Could you check a few things on this drawing? It's one solid part, dimensions in mm from its lowest x, y, z. A direction names the side the tool comes from. Give positions to 0.01 mm unless a question says otherwise; leave off trailing zeros. Use one line per item in the form item = value.
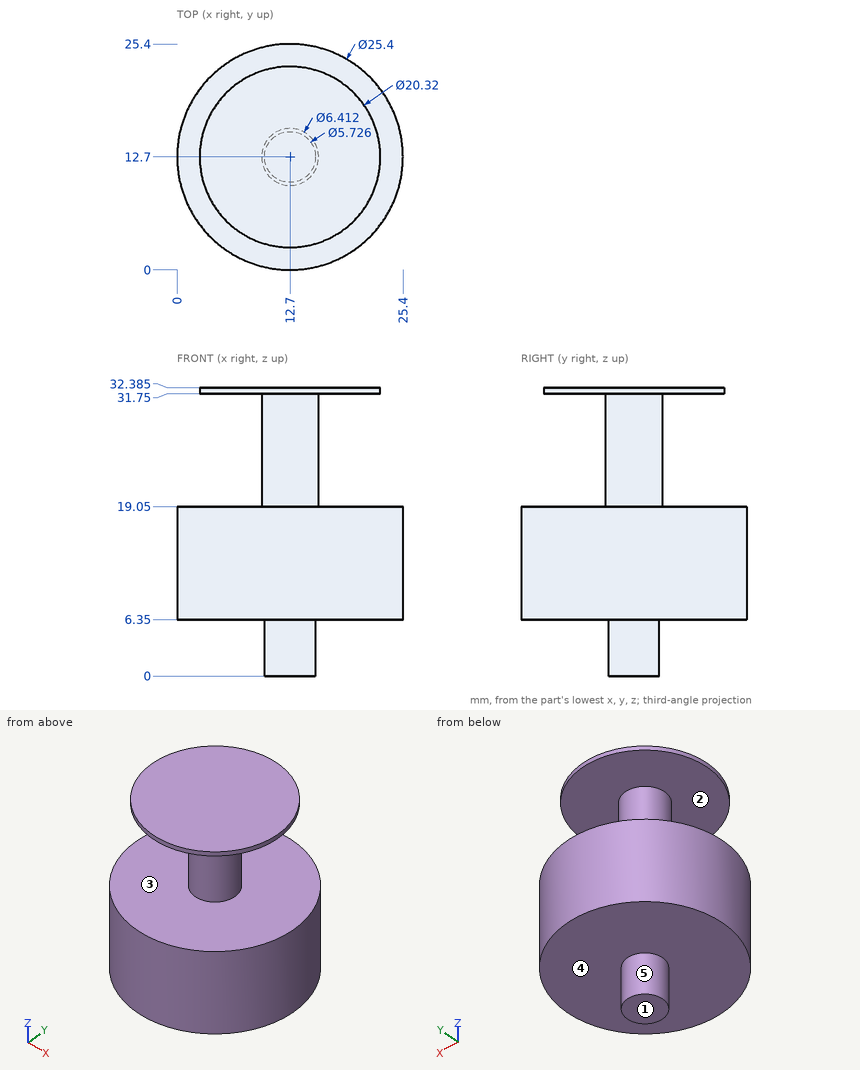
Q1. Thinking about a two-plate mould opening in Z: for the marked faces 3, 4 and 5, which applies, +Z half, -Z half, draft (parallel to the pull), parting line (faces both ways), or undercut?
Found:
face_3 = undercut
face_4 = -Z half
face_5 = draft
Q2. I'm going to push flat-ended pins straight in: pin 1 Ø1 at (y, z) = (9.5, 12.5) entering from +X; pin 2 Ø5 at (x, z) = (19, 17.5) entering from -Y; pin 3 Ø4 at (x, z) = (5, 18.5) entering from +Y. Where does each tip first touch, or does it pass through?
Found:
pin_1 = 25.11
pin_2 = 0.58
pin_3 = 24.05
Q3. I need wall thicknesses on L1, parallel to Z at x = 17, y = 6.5 (3 decimals); L2, parallel to Z at x = 17, y = 22.25; L3, parallel to Y at x = 12.5, z = 12.5. Which ranges of each line are inside material? Lowest first, please.
Found:
L1 = 6.35 to 19.05, 31.75 to 32.385
L2 = 6.35 to 19.05
L3 = 0 to 25.4
Q4. On a 3-axis mill with a long thin cutter (end or side, diameter ignored), from which of +Z, -Z, +X, -X, +Y, -Y can I reach the whole of each face in a straight line? I mean the marked faces 1 and 2. Say none if no direction works.
Found:
face_1 = -Z, +X, -X, +Y, -Y
face_2 = none
